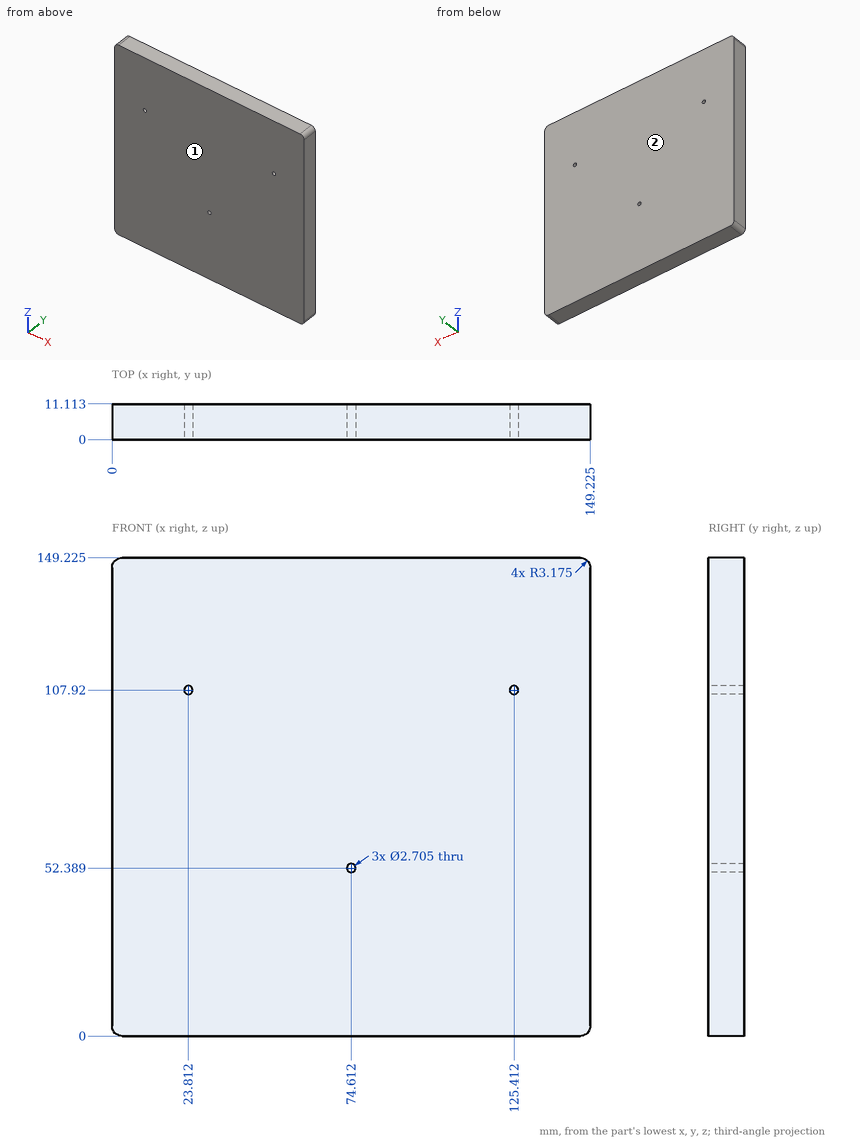
Answer from the drawing. Dimensions are ordinates in mm from the lowest x, y and z of the part. Give positions to 0.01 mm unless a question says otherwise; leave off trailing zeros. Answer as a JSON object with one key per item and string values.
1. Find the intervals of material crossed by L1, parallel to X at y = 5, z = 52 (1 decimal); L2, parallel to X at y = 7, z = 53.5 (1 decimal), in increasing order. Write a range as [from, to].
Determined:
{"L1": "[0, 73.3], [75.9, 149.2]", "L2": "[0, 73.8], [75.4, 149.2]"}
2. A flat-ended cylindrical pin translates along its axis: pin 1 Ø5 at (x, y) = (38.5, 10) entering from -Z. Find the tip coordinate at first contact, or state that the pin passes through.
Determined:
{"pin 1": "z = 0"}
3. For a pull along Y with two mould halves and no side action, classify the marked faces 1 and 2 as pulls with the +Y half, pulls with the -Y half, needs draft (parallel to the pull), parting line crosses it, or undercut.
Determined:
{"face 1": "pulls with the -Y half", "face 2": "pulls with the +Y half"}
